Geometry: final body of the model. Coordinates: model frame, mm. A direction names the side the tool comes from. Round coordinates to 2 decimals unless told otherwise and drop trailing zeros. Loops run counter-clockwise (first coordinate to the right, second up) from the corner with the lowest first, then second, coordinate; pieces in that order, holes last. Notation, with made-up numbers: (4.25, 42) -> (36.25, 42) arc R23 ccw to (36.25, 68) -> close; hole circle Ø5 at (-10.5, 17.25). An arc over 180 degrees is marked (long way). Answer in a Markdown table with one row per item.
```python
from build123d import *

# Parameters (mm, degrees)
F0_W     = 1.2
F0_H     = 1.2
F0_W_2   = 6.8
F0_H_2   = 35.5907311706
F0_H_3   = 1.2092688294
F1_DEPTH = 20
F3_DEPTH = 40.4
F4_R     = 2
F5_R     = 2.5
F6_R     = 2
F7_R     = 1


# Not quite as in the source:
# - ends of sketch curves that miss each other by under 0.0002 mm in the source are joined


with BuildPart() as f1:
    # F0 (on Right) → F1 (new body)
    with BuildSketch(Plane.YZ):
        with Locations((-0.6, 82.4221718073)):
            Rectangle(F0_W, F0_H)
        with Locations((-4.6, 82.4221718073)):
            Rectangle(F0_W_2, F0_H)
        with Locations((-0.6, 64.026806222)):
            Rectangle(F0_W, F0_H_2)
        with Locations((-0.6, 45.626806222)):
            Rectangle(F0_W, F0_H_3)
        Polygon((-1.2, 45.0221718073), (-1.2, 46.2314406367), (-10.7555877391, 46.2314406367), (-10.7812210649, 46.2314406367), (-10.8245881359, 46.2430607959), (-25.0829152046, 50.0635639224), (-31.8443964743, 51.8752954254), (-32.1549790177, 50.7161843506), (-25.393497748, 48.9044528476), (-10.9046093128, 45.0221710554), align=None)
    extrude(amount=F1_DEPTH)

    # F2 (on face) → F3 (cut)
    with BuildSketch(Plane.XY.offset(83.0221718073)):
        Polygon((7.2019821778, -9.2), (-6.1580585316, -9.2), (-6.1580585316, -39.2), (25.7106479257, -39.2), (25.7106479257, -9.2), (12.7980178222, -9.2), (12.7980178222, -35.1533853561), (7.2019821778, -35.1533853561), align=None)
    extrude(amount=-F3_DEPTH, mode=Mode.SUBTRACT)

    # F4
    f4_edges = [f1.edges().sort_by_distance(p)[0] for p in [
        (0, -9.2, 45.626806),
        (20, -9.2, 45.626806),
    ]]
    fillet(f4_edges, radius=F4_R)

    # F5
    f5_edges = [f1.edges().sort_by_distance(p)[0] for p in [
        (12.798018, -31.999688, 51.29574),
        (7.201982, -31.999688, 51.29574),
    ]]
    fillet(f5_edges, radius=F5_R)

    # F6
    f6_edges = [f1.edges().sort_by_distance(p)[0] for p in [
        (20, -8, 82.422172),
        (0, -8, 82.422172),
    ]]
    fillet(f6_edges, radius=F6_R)

    # F7
    f7_edges = [f1.edges().sort_by_distance(p)[0] for p in [
        (10, -1.2, 46.231441),
        (10, 0, 45.022172),
        (10, 0, 83.022172),
        (10, -1.2, 81.822172),
    ]]
    fillet(f7_edges, radius=F7_R)


solid = f1.part
```
Item 1: Pin query (flat end, axial travel): pin 1 Ø10 at (x, y) = (4.5, -21) entering from -Z; pin 2 Ø1.3 at (x, z) = (4, 45.5) entering from -Y; pin 3 Ø3 at (x, y) = (6.5, -12.5) entering from +Z. Return the tip coordinate at first contact, or that it passes through.
Answer:
| item | result |
|---|---|
| pin 1 | stops at z = 46.6 |
| pin 2 | stops at y = -9.2 |
| pin 3 | stops at z = 47.05 |
Item 2: Cut plane D-D (x = 1.5). Output: boundary loops of the cut face in (y, z), then the cut area to 3 significant figures.
Answer:
| item | result |
|---|---|
| outline | (-9.14, 45.02) -> (-1, 45.02) arc R1 ccw to (0, 46.02) -> (0, 82.02) arc R1 ccw to (-1, 83.02) -> (-7.94, 83.02) -> (-7.94, 81.82) -> (-2.2, 81.82) arc R1 cw to (-1.2, 80.82) -> (-1.2, 47.23) arc R1 cw to (-2.2, 46.23) -> (-9.14, 46.23) -> close |
| area | 63.3 mm² |
Item 3: Reachability of faces 4 (the face through (10, -5, 46.231)), 5 (the face through (5, -9.2, 46)), 6 (the face through (10.14, -1.501, 81.537)), 7 (the face through (15, -9.2, 46)) from +Z, -Z, +X, -X, +Y, -Y: full face, straight path, thin tool, end or side. Return the list, or none.
Answer:
| item | result |
|---|---|
| face 4 | +X, -X |
| face 5 | +Z, -Z, -X, -Y |
| face 6 | +X, -X, -Y |
| face 7 | +Z, -Z, +X, -Y |
Item 4: Cut plane C-C (y = -24.5). Output: boundary loops of the cut face in (x, z), then the cut area to 3 significant figures.
Answer:
| item | result |
|---|---|
| outline | (7.2, 48.67) -> (12.8, 48.67) -> (12.8, 49.91) -> (7.2, 49.91) -> close |
| area | 6.95 mm² |
Item 5: Draft query along Y for faces 1 (the face through (10.14, -1.49, 46.53)), 2 (the face through (10, 0, 64)), 3 (the face through (0.57, -7.4, 82.43)). Return one class per face: pulls with the +Y half, pulls with the -Y half, needs draft (parallel to the pull), parting line crosses it, or undercut.
Answer:
| item | result |
|---|---|
| face 1 | undercut |
| face 2 | pulls with the +Y half |
| face 3 | pulls with the -Y half |
Item 6: Line query: probe 1 along Z at (x, y) = (17, -7.5); probe 2 along Y at (x, z) = (8.25, 73); probe 3 along Z at (x, y) = (7.25, -25). Output: solid intervals per line, ascending. Write a range as [from, to].
Answer:
| item | result |
|---|---|
| probe 1 | z = [45.02, 46.23], [81.82, 83.02] |
| probe 2 | y = [-1.2, 0] |
| probe 3 | z = [48.8, 50.04] |
Item 7: Cut plane A-A (x = 6.5). Output: boundary loops of the cut face in (y, z).
Answer:
| item | result |
|---|---|
| outline | (-9.2, 45.02) -> (-1, 45.02) arc R1 ccw to (0, 46.02) -> (0, 82.02) arc R1 ccw to (-1, 83.02) -> (-8, 83.02) -> (-8, 81.82) -> (-2.2, 81.82) arc R1 cw to (-1.2, 80.82) -> (-1.2, 47.23) arc R1 cw to (-2.2, 46.23) -> (-9.2, 46.23) -> close |
Item 8: Cut plane B-B (z = 71). Output: boundary loops of the cut face in (x, y).
Answer:
| item | result |
|---|---|
| outline | (0, -1.2) -> (20, -1.2) -> (20, 0) -> (0, 0) -> close |
